Design review of the part shown in the three views and the two pictorial views. Dimensions are in mm from the part's minimum x, y and z. Round coordinates to 2 decimals unless told otherwise and drop trailing zeros. Loops run counter-clockwise (first coordinate to the right, second up) from the corner with the lowest first, then second, coordinate; pieces in that order, holes last. Notation, with made-up numbers: (-19, -7.75) -> (9, -7.75) arc R18 ccw to (9, 0.25) -> close; hole circle Ø3 at (38, 68). An arc over 180 degrees is marked (long way). Use a Markdown table: item, result. Add a question column.
1) Mouldability with a two-part tool opening along X and no side actions: class the marked faces 1, 2 and 3 as released by +X, released by -X, zero draft, split by the parting line, or undercut.
2) Wall thickness on probe 1 along X at (y, z) = (18.9, 2); probe 2 along X at (y, z) = (11, 0.8); probe 3 along Y at (x, z) = (14.75, 2.3): over which ranges is each line inside the solid? List them lowest first.
3) Consider section C-C on y = 8.75. Give the boundary of the cut face in (x, z).
4) Consider section D-D on z = 1.25. Give the boundary of the cut face in (x, y), plus the area to 3 significant figures.
5) Consider section B-B on x = 16.25. Give the boundary of the cut face in (y, z).
6) Insertion check: pin 1 (6 mm diameter, centred on x = 15, y = 13.5, fed in from -Z); pin 2 (1 mm diameter, centred on y = 4, z = 1, fed in from +X). Each pin has a flat end and moves straight along its axis. Give the tip position at first contact, or say it passes through.
7) Consider section A-A on z = 2.4. Give the boundary of the cut face in (x, y), plus the area to 3 significant figures.
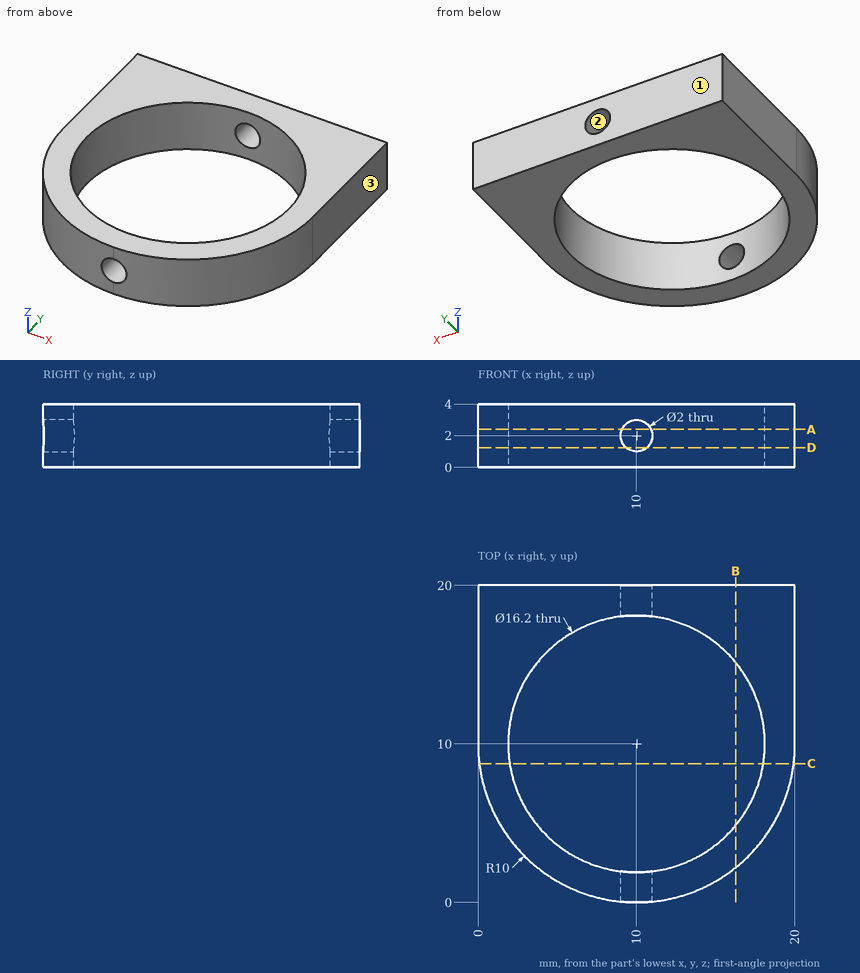
Result set:
| question | item | result |
|---|---|---|
| 1 | face 1 | zero draft |
| 1 | face 2 | undercut |
| 1 | face 3 | released by +X |
| 2 | probe 1 | 0 to 9, 11 to 20 |
| 2 | probe 2 | 0 to 1.96, 18.04 to 20 |
| 2 | probe 3 | 1.2 to 3.44, 16.56 to 20 |
| 3 | outline | (0.08, 0) -> (2, 0) -> (2, 4) -> (0.08, 4) -> close; (18, 0) -> (19.92, 0) -> (19.92, 4) -> (18, 4) -> close |
| 4 | outline | (0, 10) arc R10 ccw to (9.34, 0.02) -> (9.34, 1.93) arc R8.1 cw to (9.34, 18.07) -> (9.34, 20) -> (0, 20) -> close; (10.66, 0.02) arc R10 ccw to (20, 10) -> (20, 20) -> (10.66, 20) -> (10.66, 18.07) arc R8.1 cw to (10.66, 1.93) -> close |
| 4 | area | 146 mm2 |
| 5 | outline | (2.19, 0) -> (4.85, 0) -> (4.85, 4) -> (2.19, 4) -> close; (15.15, 0) -> (20, 0) -> (20, 4) -> (15.15, 4) -> close |
| 6 | pin 1 | z = 0 |
| 6 | pin 2 | x = 18.35 |
| 7 | outline | (0, 10) arc R10 ccw to (9.08, 0.04) -> (9.08, 1.95) arc R8.1 cw to (9.08, 18.05) -> (9.08, 20) -> (0, 20) -> close; (10.92, 0.04) arc R10 ccw to (20, 10) -> (20, 20) -> (10.92, 20) -> (10.92, 18.05) arc R8.1 cw to (10.92, 1.95) -> close |
| 7 | area | 144 mm2 |
